Work out the finished part from the listing and answer in its coordinate system (mm). Round coordinates to 2 decimals unless told otherwise and drop trailing zeros. Order: outer loops, then holes, each group sorted by start corner. A loop starts at its lowest first (then second) coordinate and runs counter-clockwise, first axis right, second up. Notation, with made-up numbers: M 78.5,41.25 L 93.5,41.25 A28 ccw 93.5,59.25 Z; hole C 35,51 d9. An arc over 180 degrees is marked long. Return JSON: item names as keys, results as strings.
from build123d import *

# Parameters (mm, degrees)
SKETCH1_W            = 25.4
SKETCH1_H            = 45
BOSS_EXTRUDE1_DEPTH  = 6
FILLET1_R            = 4
M5_CLEARANCE_HOLE1_D = 5.5
M5_CLEARANCE_HOLE2_D = 5.5


with BuildPart() as part:
    # Sketch1 → Boss-Extrude1 (new body, symmetric)
    with BuildSketch(Plane.XY):
        Rectangle(SKETCH1_W, SKETCH1_H)
    extrude(amount=BOSS_EXTRUDE1_DEPTH, both=True)

    # Fillet1
    fillet1_edges = [part.edges().sort_by_distance(p)[0] for p in [
        (-12.7, 22.5, 0),
        (12.7, 22.5, 0),
        (12.7, -22.5, 0),
        (-12.7, -22.5, 0),
    ]]
    fillet(fillet1_edges, radius=FILLET1_R)

    # M5 Clearance Hole1 (through all)
    with Locations(Plane.ZY.offset(12.7)):
        with Locations((0, 0)):
            Hole(M5_CLEARANCE_HOLE1_D / 2)

    # M5 Clearance Hole2 (through all)
    with Locations(Plane(origin=(0, 0, -6), x_dir=(-1, 0, 0), z_dir=(0, 0, -1))):
        with Locations((0, 12.5), (0, -12.5)):
            Hole(M5_CLEARANCE_HOLE2_D / 2)


solid = part.part
Item 1: Find section D-D (z = -4.5). Determine the outline of the cut face in (x, y).
Output:
{"outline": "M -12.7,-18.5 A4 ccw -8.7,-22.5 L 8.7,-22.5 A4 ccw 12.7,-18.5 L 12.7,18.5 A4 ccw 8.7,22.5 L -8.7,22.5 A4 ccw -12.7,18.5 Z; hole C 0,-12.5 d5.5; hole C 0,12.5 d5.5"}
Item 2: Find section C-C (y = 0). Determine the outline of the cut face in (x, z).
Output:
{"outline": "M -12.7,-6 L 12.7,-6 L 12.7,-2.75 L -12.7,-2.75 Z; M -12.7,2.75 L 12.7,2.75 L 12.7,6 L -12.7,6 Z"}
Item 3: Find section B-B (x = 0). Determine the outline of the cut face in (y, z).
Output:
{"outline": "M -22.5,-6 L -15.25,-6 L -15.25,6 L -22.5,6 Z; M -9.75,-6 L 9.75,-6 L 9.75,6 L -9.75,6 Z; M 15.25,-6 L 22.5,-6 L 22.5,6 L 15.25,6 Z; hole C 0,0 d5.5"}
Item 4: This flat-tipped pin is pushed along its axis until it touches: pin 1 (1 mm diameter, centred on x = 10, z = 3.5, fed in from -Y). Where does it stop, or does it pass through?
Output:
{"pin 1": "stops at y = -22.42"}
Item 5: Find section A-A (z = 0). Determine the outline of the cut face in (x, y).
Output:
{"outline": "M -12.7,-18.5 A4 ccw -8.7,-22.5 L 8.7,-22.5 A4 ccw 12.7,-18.5 L 12.7,-2.75 L -12.7,-2.75 Z; M -12.7,2.75 L 12.7,2.75 L 12.7,18.5 A4 ccw 8.7,22.5 L -8.7,22.5 A4 ccw -12.7,18.5 Z; hole C 0,-12.5 d5.5; hole C 0,12.5 d5.5"}
Item 6: Consider line 1 along Y through (x, z) = (0, 3); line 2 along Y through (x, z) = (-2.25, 5.5); line 3 along Y through (x, z) = (1.75, 0). Determine where each line is inside the solid, lowest interval first. Write a range as [from, to].
Output:
{"line 1": "y = [-22.5, -15.25], [-9.75, 9.75], [15.25, 22.5]", "line 2": "y = [-22.5, -14.08], [-10.92, 10.92], [14.08, 22.5]", "line 3": "y = [-22.5, -14.62], [-10.38, -2.75], [2.75, 10.38], [14.62, 22.5]"}
Item 7: The mould has two halves that part along X. Classify faces 1 (the cylindrical face through (-2.027, 14.359, 0.084)), 2 (the flat face through (0, -22.5, 0)), 3 (the flat face through (-12.7, 0, 3)): pulls with the +X half, pulls with the -X half, needs draft (parallel to the pull), parting line crosses it, or undercut.
Output:
{"face 1": "undercut", "face 2": "needs draft", "face 3": "pulls with the -X half"}
